from build123d import *

# Parameters (mm, degrees)
SKETCH_1_W                      = 70
SKETCH_1_H                      = 118
EXTRUDE_1_DEPTH                 = 5
CUT_EXTRUDE_1_REACH             = 70.782
SKETCH_2_W                      = 5
SKETCH_2_H                      = 20
CUT_EXTRUDE_1_DIRECTION_2_DEPTH = 69.782265156
PATTERN_LINEAR_1_COUNT          = 3
PATTERN_LINEAR_1_PITCH          = 40
CUT_EXTRUDE_3_REACH             = 70.782
SKETCH_4_W                      = 5
SKETCH_4_H                      = 20
PATTERN_LINEAR_4_COUNT          = 3
PATTERN_LINEAR_4_PITCH          = 40
SKETCH_3_W                      = 20
SKETCH_3_H                      = 5
EXTRUDE_2_DEPTH                 = 5
PATTERN_LINEAR_5_COUNT          = 2
PATTERN_LINEAR_5_PITCH          = 40


with BuildPart() as part:
    # 스케치1 → 보스-돌출1 (new body)
    with BuildSketch(Plane.XY):
        Rectangle(SKETCH_1_W, SKETCH_1_H)
    extrude(amount=EXTRUDE_1_DEPTH)

    # 스케치2 → 컷-돌출1 (cut, up to next)
    with BuildSketch(Plane.XY.offset(5), mode=Mode.PRIVATE) as cut_extrude_1_sk1:
        with Locations((-32.5, -49)):
            Rectangle(SKETCH_2_W, SKETCH_2_H)
    cut_extrude_1_tool1 = extrude(cut_extrude_1_sk1.sketch, amount=-CUT_EXTRUDE_1_REACH, mode=Mode.PRIVATE) & part.part
    cut_extrude_1 = cut_extrude_1_tool1.solids().sort_by_distance((-32.5, -49, 5))[0]
    add(cut_extrude_1, mode=Mode.SUBTRACT)

    # 스케치2 → 컷-돌출1 direction 2 (cut)
    with BuildSketch(Plane.XY.offset(5)):
        with Locations((-32.5, -49)):
            Rectangle(SKETCH_2_W, SKETCH_2_H)
    cut_extrude_1_direction_2 = extrude(amount=CUT_EXTRUDE_1_DIRECTION_2_DEPTH, mode=Mode.SUBTRACT)

    # 선형 패턴1: 컷-돌출1, 컷-돌출1 direction 2 ×3
    with Locations(*[(0, i * PATTERN_LINEAR_1_PITCH, 0) for i in range(1, PATTERN_LINEAR_1_COUNT)]):
        add(cut_extrude_1, mode=Mode.SUBTRACT)
        add(cut_extrude_1_direction_2, mode=Mode.SUBTRACT)

    # 스케치4 → 컷-돌출3 (cut, up to next)
    with BuildSketch(Plane.XY.offset(5), mode=Mode.PRIVATE) as cut_extrude_3_sk1:
        with Locations((32.5, -49)):
            Rectangle(SKETCH_4_W, SKETCH_4_H)
    cut_extrude_3_tool1 = extrude(cut_extrude_3_sk1.sketch, amount=-CUT_EXTRUDE_3_REACH, mode=Mode.PRIVATE) & part.part
    cut_extrude_3 = cut_extrude_3_tool1.solids().sort_by_distance((32.5, -49, 5))[0]
    add(cut_extrude_3, mode=Mode.SUBTRACT)

    # 선형 패턴4: 컷-돌출3 ×3
    with Locations(*[(0, i * PATTERN_LINEAR_4_PITCH, 0) for i in range(1, PATTERN_LINEAR_4_COUNT)]):
        add(cut_extrude_3, mode=Mode.SUBTRACT)

    # 스케치3 → 보스-돌출2 (add)
    with BuildSketch(Plane.XY.offset(5)):
        with Locations((-25, 61.5)):
            Rectangle(SKETCH_3_W, SKETCH_3_H)
    extrude_2 = extrude(amount=-EXTRUDE_2_DEPTH)

    # 선형 패턴5: 보스-돌출2 ×2
    with Locations(*[(i * PATTERN_LINEAR_5_PITCH, 0, 0) for i in range(1, PATTERN_LINEAR_5_COUNT)]):
        add(extrude_2)


solid = part.part
The listing builds one solid part. Answer for the finished solid, in the listing's coordinates (mm). A direction names the side the tool comes from. Round coordinates to 2 decimals unless told otherwise and drop trailing zeros. Order: outer loops, then holes, each group sorted by start corner. A loop starts at its lowest first (then second) coordinate and runs counter-clockwise, first axis right, second up. Notation, with made-up numbers: (70, 51.5) -> (124, 51.5) arc R26 ccw to (124, 66.5) -> close; hole circle Ø11 at (45.5, 5). An arc over 180 degrees is marked (long way). Write each question's results on one line, items separated by ' | '. Start each with the question number.
Q1. Find section C-C (x = -10). Determine the outline of the cut face in (y, z), then the cut area to 3 significant figures.
Q2. Each of these flat-tipped pins is pushed along its axis until it touches: pin 1 (2.5 mm diameter, centred on x = 29.5, z = 1.5, fed in from +Y); pin 2 (1.5 mm diameter, centred on x = -31.5, z = 3, fed in from -Y); pin 3 (2.5 mm diameter, centred on y = -44, z = 3, fed in from +X). Where does it stop, or does it pass through?
Q3. The mould has two halves that part along X. Classify faces 1 (the flat face through (-35, -29, 2)), 2 (the flat face through (35, 11, 2)), 3 (the flat face through (-5, 59, 2)), 4 (the flat face through (0, 3, 5)): pulls with the +X half, pulls with the -X half, needs draft (parallel to the pull), parting line crosses it, or undercut.
Q4. Straight lines are drawn through the part: probe 1 along Y at (x, z) = (-31, 1.4); probe 2 along Y at (x, z) = (26, 1.05); probe 3 along X at (y, z) = (-15, 3.5). For each, find the intervals that lie inside material, in ascending order. Write a range as from..to.
Q5. Find section B-B (y = -6). Determine the outline of the cut face in (x, z), then the cut area to 3 significant figures.
Q6. Which of the six approach directions +Z, -Z, +X, -X, +Y, -Y give full straight-line access (tool end or side, diameter ignored) to faces 5 (the flat face through (-33, 41, 3)), 6 (the flat face through (32, -39, 3)), 7 (the flat face through (30, 59, 2))?
Worked answers:
1) outline: (-59, 0) -> (59, 0) -> (59, 5) -> (-59, 5) -> close | area: 590 mm2
2) pin 1: stops at y = 59 | pin 2: stops at y = -39 | pin 3: stops at x = 30
3) face 1: pulls with the -X half | face 2: pulls with the +X half | face 3: undercut | face 4: needs draft
4) probe 1: y = -39..-19, 1..21, 41..64 | probe 2: y = -59..59 | probe 3: x = -30..30
5) outline: (-30, 0) -> (30, 0) -> (30, 5) -> (-30, 5) -> close | area: 300 mm2
6) face 5: +Z, -Z, -X | face 6: +Z, -Z, +X, -Y | face 7: +Z, -Z, +X, +Y
